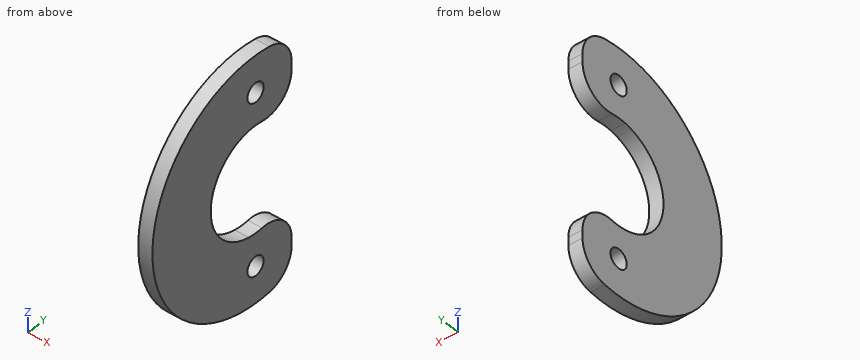
Autodesk Inventor part; units mm, degrees
ref_plane "YZ Plane" through (0, 0, 0) normal (1, 0, 0) x (0, 1, 0)
ref_plane "XZ Plane" through (0, 0, 0) normal (0, 1, 0) x (-1, 0, 0)
ref_plane "XY Plane" through (0, 0, 0) normal (0, 0, 1) x (1, 0, 0)
ref_plane "Work Plane1" through (-214.9581, 261.0384, -210.6802) normal (1, 0, 0) x (0, 1, 0)
sketch "Sketch1" plane through (-214.9581, 261.0384, -210.6802) normal (1, 0, 0) x (0, 1, 0)
  arc A0 (-304.8, -19.05) -> (-298.45, -25.4) centre (-298.45, -19.05) ccw
  line L0 (-298.45, -25.4) -> (304.8, -25.4)
  line L1 (304.8, -25.4) -> (304.8, 25.4)
  line L2 (304.8, 25.4) -> (-298.45, 25.4)
  arc A1 (-298.45, 25.4) -> (-304.8, 19.05) centre (-298.45, 19.05) ccw
  line L3 (-304.8, 19.05) -> (-304.8, 17.2126)
  arc A2 (-304.8, 17.2126) -> (-297.523, 10.9306) centre (-298.45, 17.2126) ccw
  arc A3 (-297.523, -10.9306) -> (-297.523, 10.9306) centre (-295.91, 0) ccw
  arc A4 (-297.523, -10.9306) -> (-304.8, -17.2126) centre (-298.45, -17.2126) ccw
  line L4 (-304.8, -17.2126) -> (-304.8, -19.05)
  circle A5 centre (-295.91, 17.78) radius 2
  circle A6 centre (-295.91, -17.78) radius 2
  circle A7 centre (292.1, 12.7) radius 2
  circle A8 centre (292.1, -12.7) radius 2
  circle A9 centre (266.7, 12.7) radius 2
  circle A10 centre (266.7, -12.7) radius 2
  circle A11 centre (-295.91, 0) radius 11.049
  circle A12 centre (-295.91, 0) radius 25.4
  line L5 (-287.02, 23.7934) -> (-287.02, -23.7934)
  point P0 (-261.0384, 210.6802)
  point P1 (-287.02, 6.5611)
  point P2 (-287.02, -6.5611)
  point P3 (-297.523, -10.9306)
  dimension "d0" = 17.78
extrude "Extrusion1" add sketch "Sketch1" along normal blind 3 contours L4 A4 A3 L5 A12 A0 | A0 A12 A1 L3 A2 A11 A4 L4 | A12 L5 A3 A2 L3 A1
fillet "Fillet1" radius 6.35 4 edges at (-213.4581, -25.9816, -186.8868) (-213.4581, -25.9816, -217.2413) (-213.4581, -25.9816, -204.1191) (-213.4581, -25.9816, -234.4736)
properties part number "DropBarJoint"
Input: part model. Units: mm. Frame: model coordinates. Round coordinates to 2 decimals unless told otherwise and drop trailing zeros. Order: outer loops, then holes, each group sorted by start corner. A loop starts at its lowest first (then second) coordinate and runs counter-clockwise, first axis right, second up. Notation, with made-up numbers: (11, -0.5) - (70, -0.5) arc R26 cw to (70, 22.5) - close; hole circle Ø11 at (82.5, -15). An arc over 180 degrees is marked (long way). Answer as a JSON object with one key per item and string values. Group by question number.
(1) Cut plane C-C (y = -38.5). Return loops of the section in (x, z), then the cut area to 3 significant figures.
(2) Cut plane A-A (y = -35). Return loops of the section in (x, z), then the cut area to 3 significant figures.
(3) Material intervals for probe 1 along Z at (x, y) = (-214.7, -29.5); probe 2 along Z at (x, y) = (-212.6, -37.5); probe 3 along Z at (x, y) = (-213, -47), sorted ascending. Write a range as from..to.
(4) Pin query (flat end, axial travel): P1, Ø1.5, axis at x = -213.5, y = -48, coming from the -Z side; P2, Ø1.5, axis at x = -212.5, y = -35, coming from the +Z side; P3, Ø3, axis at y = -34.87, z = -228.46, coming from the -X side; P4, Ø1, axis at x = -213.5, y = -51.5, coming from the +Z side. Return the tip coordinate at first contact, or that it passes through.
(5) Cut plane D-D (z = -220.5). Return loops of the section in (x, y).
Here are the results:
{
 "1": {"outline": "(-214.96, -235.82) - (-211.96, -235.82) - (-211.96, -221.12) - (-214.96, -221.12) - close; (-214.96, -200.24) - (-211.96, -200.24) - (-211.96, -185.54) - (-214.96, -185.54) - close", "area": "88.2 mm^2"},
 "2": {"outline": "(-214.96, -236.08) - (-211.96, -236.08) - (-211.96, -230.46) - (-214.96, -230.46) - close; (-214.96, -226.46) - (-211.96, -226.46) - (-211.96, -221.73) - (-214.96, -221.73) - close; (-214.96, -199.63) - (-211.96, -199.63) - (-211.96, -194.9) - (-214.96, -194.9) - close; (-214.96, -190.9) - (-211.96, -190.9) - (-211.96, -185.28) - (-214.96, -185.28) - close", "area": "62.2 mm^2"},
 "3": {"probe 1": "z = -235.24..-222.21, -199.15..-186.12", "probe 2": "z = -235.94..-221.41, -199.95..-185.42", "probe 3": "z = -233..-188.36"},
 "4": {"P1": "stops at z = -232.86", "P2": "stops at z = -185.28", "P3": "passes through", "P4": "stops at z = -191.06"},
 "5": {"outline": "(-214.96, -58.3) - (-211.96, -58.3) - (-211.96, -39.94) - (-214.96, -39.94) - close"}
}
